from build123d import *

# Parameters (mm, degrees)
BOSS_EXTRUDE1_DEPTH         = 5
BOSS_EXTRUDE2_DEPTH         = 6
FILLET1_R                   = 1.3
M3_TAPPED_HOLE1_D           = 2.5
M3_TAPPED_HOLE1_CSINK_D     = 3.05
M3_TAPPED_HOLE1_CSINK_ANGLE = 90


with BuildPart() as part:
    # Sketch1 → Boss-Extrude1 (new body)
    with BuildSketch(Plane(origin=(0, 0, 0), x_dir=(1, 0, 0), z_dir=(0, 1, 0))):
        with BuildLine():
            Line((-4.5, 0), (-4.5, 10))
            ThreePointArc((-4.5, 10), (0, 12.044483976), (4.5, 10))
            Line((4.5, 10), (4.5, 0))
            ThreePointArc((4.5, 0), (0, -2.044483976), (-4.5, 0))
        make_face()
    extrude(amount=BOSS_EXTRUDE1_DEPTH)

    # Sketch2 → Boss-Extrude2 (add)
    with BuildSketch(Plane(origin=(0, 5, 0), x_dir=(1, 0, 0), z_dir=(0, 1, 0))):
        with BuildLine():
            Line((-2.692561773, 11.403358064), (-2.692561773, -1.403358064))
            ThreePointArc((-2.692561773, -1.403358064), (-3.66409466, -0.78901897), (-4.5, 0))
            Line((-4.5, 0), (-4.5, 10))
            ThreePointArc((-4.5, 10), (-3.66409466, 10.78901897), (-2.692561773, 11.403358064))
        make_face()
        with BuildLine():
            Line((4.5, 10), (4.5, 0))
            ThreePointArc((4.5, 0), (3.66409466, -0.78901897), (2.692561773, -1.403358064))
            Line((2.692561773, -1.403358064), (2.692561773, 11.403358064))
            ThreePointArc((2.692561773, 11.403358064), (3.66409466, 10.78901897), (4.5, 10))
        make_face()
    extrude(amount=BOSS_EXTRUDE2_DEPTH)

    # Fillet1
    fillet1_edges = [part.edges().sort_by_distance(p)[0] for p in [
        (-3.66409466, 11, -10.78901897),
        (-3.66409466, 11, 0.78901897),
        (3.66409466, 11, -10.78901897),
        (3.66409466, 11, 0.78901897),
    ]]
    fillet(fillet1_edges, radius=FILLET1_R)

    # M3 Tapped Hole1 (through all)
    with Locations(Plane(origin=(4.5, 0, 0), x_dir=(0, 0, -1), z_dir=(1, 0, 0))):
        with Locations((5, 8.818847832)):
            CounterSinkHole(M3_TAPPED_HOLE1_D / 2, M3_TAPPED_HOLE1_CSINK_D / 2, counter_sink_angle=M3_TAPPED_HOLE1_CSINK_ANGLE)


solid = part.part
Design review of the part built by this model. Coordinates are the model's own, in mm. A direction names the side the tool comes from. Coordinates: 2 decimals unless noted, no trailing zeros. Order: outer loops, then holes, each group sorted by start corner. A loop starts at its lowest first (then second) coordinate and runs counter-clockwise, first axis right, second up. Notation, with made-up numbers: M 17,-16 L 37,-16 A21 cw 37,-2 Z; hole C -14.75,11 d10. An arc over 180 degrees is marked long. Use a Markdown table: item, result.
(1) Draft analysis for pull direction X (two halves, no side actions). For faces 3 (the flat face through (-4.5, 5, -5)), 4 (the flat face through (2.693, 7, -5)), 5 (the flat face through (4.5, 5, -5)), state which applies: released by +X, released by -X, zero draft, split by the parting line, or undercut.
Worked answers:
| item | result |
|---|---|
| face 3 | released by -X |
| face 4 | undercut |
| face 5 | released by +X |
(2) Wall thickness on probe 1 along Y at (x, z) = (-3.85, -5); probe 2 along X at (y, z) = (5.75, -2); probe 3 along Y at (x, z) = (0, -9.5): over which ranges is each line inside the solid? List them lowest first.
Worked answers:
| item | result |
|---|---|
| probe 1 | y = 0 to 7.57, 10.07 to 11 |
| probe 2 | x = -4.5 to -2.69, 2.69 to 4.5 |
| probe 3 | y = 0 to 5 |
(3) Add section D-D (x = -1.75). Give the boundary of the cut face in (y, z), then the cut area to 3 significant figures.
Worked answers:
| item | result |
|---|---|
| outline | M 0,-11.78 L 5,-11.78 L 5,1.78 L 0,1.78 Z |
| area | 67.8 mm2 |
(4) Add section B-B (y = 6.75). Give the boundary of the cut face in (x, z).
Worked answers:
| item | result |
|---|---|
| outline | M -4.5,-10 A5.97 ccw -2.69,-11.4 L -2.69,1.4 A5.97 ccw -4.5,0 Z; M 2.69,-11.4 A5.97 ccw 4.5,-10 L 4.5,0 A5.97 ccw 2.69,1.4 Z |
(5) Add section C-C (y = 3.5). Give the boundary of the cut face in (x, z).
Worked answers:
| item | result |
|---|---|
| outline | M -4.5,-10 A5.97 ccw 4.5,-10 L 4.5,0 A5.97 ccw -4.5,0 Z |
(6) For faces 1 (the flat face through (-3, 11, -5)), 2 (the flat face through (-2.693, 7, -5)), list the 3-axis set-ups (+Z, -Z, +X, -X, +Y, -Y) from which the entire face can be reached by the end or side of a thin tool; tool diameter is ignored.
Worked answers:
| item | result |
|---|---|
| face 1 | +Z, -Z, +X, -X, +Y |
| face 2 | +Z, -Z, +Y |
(7) For P1, Ø3, axis at x = 1.5, y = 9.5, coming from the +Z side; P2, Ø1.6, axis at x = -0.5, z = -7.5, coming from the +Y side, all flat-tipped, find the tip position at first contact; note any pin that passes through.
Worked answers:
| item | result |
|---|---|
| P1 | stops at z = 1.4 |
| P2 | stops at y = 5 |
(8) Add section A-A (z = -5). Give the boundary of the cut face in (x, y) (3 decimals), then the cut area to 3 significant figures.
Worked answers:
| item | result |
|---|---|
| outline | M -4.5,0 L 4.5,0 L 4.5,7.294 L 4.225,7.569 L 2.693,7.569 L 2.693,5 L -2.693,5 L -2.693,7.569 L -4.5,7.569 Z; M -4.5,10.069 L -2.693,10.069 L -2.693,11 L -4.5,11 Z; M 2.693,10.069 L 4.225,10.069 L 4.5,10.344 L 4.5,11 L 2.693,11 Z |
| area | 57.6 mm2 |
